Check sheet for the modelled part. Datum: model origin and axes. Units: mm. Face numbers are marked on the shaded views. Coordinates: 2 decimals unless noted, no trailing zeros. Write each loop counter-clockwise with the first axis right and the second up, starting at its lowest first coordinate (ties: lowest second). Pieces come first, ordered by that corner, then holes. Notation, with made-up numbers: (16.25, 77) -> (56.25, 77) arc R6 ccw to (56.25, 82) -> close; hole circle Ø9 at (57.5, 34). An arc over 180 degrees is marked (long way). One line per item, written item: value. Start each with the question number.
1) Gauge pin test, flat ends, axial feed: P1, Ø1, axis at x = 14.5, y = -13, coming from the +Z side; P2, Ø12, axis at y = -8, z = -18, coming from the +X side; P3, Ø1.5, axis at x = -11, y = -14.5, coming from the +Z side. Record the tip position at first contact, or that the pin passes through.
2) Draft check along X on the marked faces 1, 2 and 3. Enter one of: +X half, -X half, draft (parallel to the pull), parting line (faces both ways), or undercut.
3) Sectioned sample at D-D on y = -22.5. Enter the section's corners in (x, z), plus the area to 3 significant figures.
4) Scan lines: line 1 along Z through (x, y) = (0, -6); line 2 along Z through (x, y) = (7.5, -22.75); line 3 along X through (y, z) = (-12.25, 3). Record each from-to range of solid material in increasing order. Write a range as [from, to].
5) Sectioned sample at A-A on x = 0. Enter the section's corners in (y, z), plus the area to 3 significant figures.
6) Sectioned sample at B-B on z = 0. Enter the section's corners in (x, y).
7) Sectioned sample at C-C on y = -5.75. Enter the section's corners in (x, z), plus the area to 3 significant figures.
```python
from build123d import *

# Parameters (mm, degrees)
F0_R     = 25.4
F1_DEPTH = 25.4
F2_R     = 12.7
F3_DEPTH = 25.401
F4_R     = 5.08


with BuildPart() as f1:
    # F0 (on Front) → F1 (new body)
    with BuildSketch(Plane.XZ):
        Circle(F0_R)
    extrude(amount=F1_DEPTH)

    # F2 (on face) → F3 (cut, through all)
    with BuildSketch(Plane.XZ.offset(25.4)):
        Circle(F2_R)
    extrude(amount=-F3_DEPTH, mode=Mode.SUBTRACT)

    # F4
    f4_edges = [f1.edges().sort_by_distance(p)[0] for p in [
        (-25.4, -25.4, 0),
        (-12.7, -25.4, 0),
    ]]
    fillet(f4_edges, radius=F4_R)


solid = f1.part
```
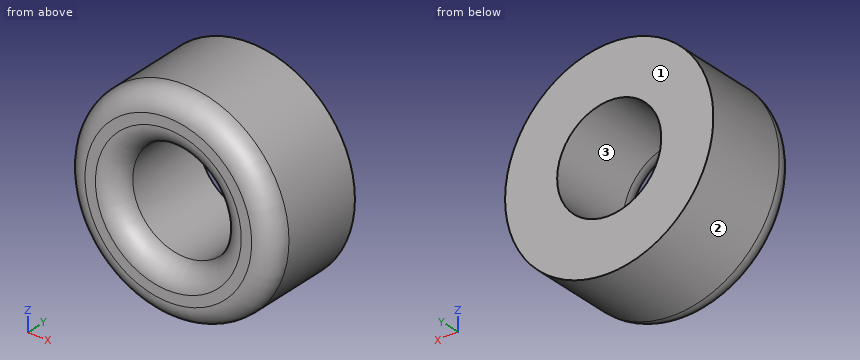
Answers:
1. P1: stops at z = 21.19
1. P2: stops at x = 22.39
1. P3: stops at z = 23.24
2. face 1: draft
2. face 2: parting line
2. face 3: undercut
3. outline: circle Ø49.82 at (0, 0); hole circle Ø26.38 at (0, 0)
3. area: 1,400 mm2
4. line 1: z = [-25.4, -12.7], [12.7, 25.4]
4. line 2: z = [-23.62, -11.01], [11.01, 23.62]
4. line 3: x = [-25.22, -12.34], [12.34, 25.22]
5. outline: (-25.4, -20.32) arc R5.08 ccw to (-20.32, -25.4) -> (0, -25.4) -> (0, -12.7) -> (-20.32, -12.7) arc R5.08 ccw to (-25.4, -17.78) -> close; (-25.4, 17.78) arc R5.08 ccw to (-20.32, 12.7) -> (0, 12.7) -> (0, 25.4) -> (-20.32, 25.4) arc R5.08 ccw to (-25.4, 20.32) -> close
5. area: 623 mm2
6. outline: (-25.4, -20.32) arc R5.08 ccw to (-20.32, -25.4) -> (-17.78, -25.4) arc R5.08 ccw to (-12.7, -20.32) -> (-12.7, 0) -> (-25.4, 0) -> close; (12.7, -20.32) arc R5.08 ccw to (17.78, -25.4) -> (20.32, -25.4) arc R5.08 ccw to (25.4, -20.32) -> (25.4, 0) -> (12.7, 0) -> close
7. outline: circle Ø50.8 at (0, 0); hole circle Ø25.4 at (0, 0)
7. area: 1,520 mm2
